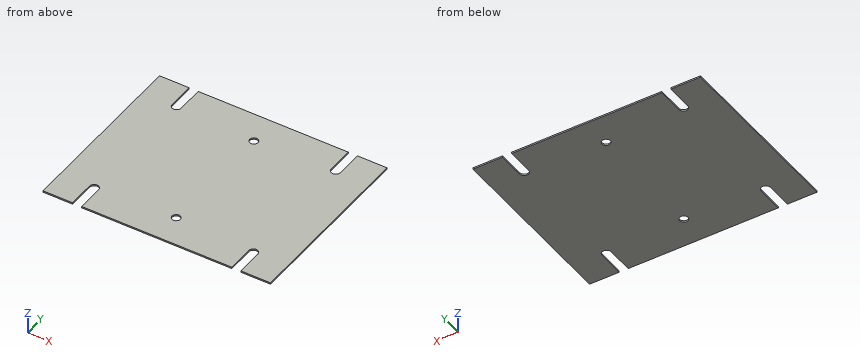
from build123d import *

# Parameters (mm, degrees)
SKETCH1_R               = 5.5
SKETCH1_R_2             = 3.25
BOSS_EXTRUDE1_DEPTH     = 2
CUT_EXTRUDE1_DEPTH      = 319.029152687
CUT_EXTRUDE1_DEPTH_BACK = 319.029152687
SKETCH2_W               = 30
SKETCH2_H               = 70
CUT_EXTRUDE2_DEPTH      = 319.029152687
CUT_EXTRUDE2_DEPTH_BACK = 319.029152687
SKETCH3_W               = 30
SKETCH3_H               = 70


with BuildPart() as part:
    # Sketch1 → Boss-Extrude1 (new body)
    with BuildSketch(Plane.XY):
        with BuildLine():
            Line((68.948821818, -26.633764286), (98.948821818, -26.633764286))
            Line((98.948821818, -26.633764286), (98.948821818, -96.633764286))
            Line((98.948821818, -96.633764286), (68.948821818, -96.633764286))
            Line((68.948821818, -96.633764286), (68.948821818, -181.633764286))
            Line((68.948821818, -181.633764286), (29.948821818, -181.633764286))
            Line((29.948821818, -181.633764286), (29.948821818, -146.633764286))
            ThreePointArc((29.948821818, -146.633764286), (23.948821818, -140.633764286), (17.948821818, -146.633764286))
            Line((17.948821818, -146.633764286), (17.948821818, -181.633764286))
            Line((17.948821818, -181.633764286), (-180.051178182, -181.633764286))
            Line((-180.051178182, -181.633764286), (-180.051178182, -146.633764286))
            ThreePointArc((-180.051178182, -146.633764286), (-186.051178182, -140.633764286), (-192.051178182, -146.633764286))
            Line((-192.051178182, -146.633764286), (-192.051178182, -181.633764286))
            Line((-192.051178182, -181.633764286), (-231.051178182, -181.633764286))
            Line((-231.051178182, -181.633764286), (-231.051178182, -100.179856115))
            Line((-231.051178182, -100.179856115), (-261.051178182, -100.179856115))
            Line((-261.051178182, -100.179856115), (-261.051178182, -30.179856115))
            Line((-261.051178182, -30.179856115), (-231.051178182, -30.179856115))
            Line((-231.051178182, -30.179856115), (-231.051178182, 58.366235714))
            Line((-231.051178182, 58.366235714), (-192.051178182, 58.366235714))
            Line((-192.051178182, 58.366235714), (-192.051178182, 23.366235714))
            ThreePointArc((-192.051178182, 23.366235714), (-186.051178182, 17.366235714), (-180.051178182, 23.366235714))
            Line((-180.051178182, 23.366235714), (-180.051178182, 58.366235714))
            Line((-180.051178182, 58.366235714), (17.948821818, 58.366235714))
            Line((17.948821818, 58.366235714), (17.948821818, 23.366235714))
            ThreePointArc((17.948821818, 23.366235714), (23.948821818, 17.366235714), (29.948821818, 23.366235714))
            Line((29.948821818, 23.366235714), (29.948821818, 58.366235714))
            Line((29.948821818, 58.366235714), (68.948821818, 58.366235714))
            Line((68.948821818, 58.366235714), (68.948821818, -26.633764286))
        make_face()
        with Locations((-81.051178182, -141.633764286)):
            Circle(SKETCH1_R, mode=Mode.SUBTRACT)
        with Locations((-81.051178182, 18.366235714)):
            Circle(SKETCH1_R, mode=Mode.SUBTRACT)
        with Locations((83.948821818, -61.633764286)):
            Circle(SKETCH1_R_2, mode=Mode.SUBTRACT)
        with Locations((-246.051178182, -65.179856115)):
            Circle(SKETCH1_R_2, mode=Mode.SUBTRACT)
    extrude(amount=BOSS_EXTRUDE1_DEPTH)

    # Sketch2 → Cut-Extrude1 (cut, two sides: drawn at the far end of the back side and taken through both)
    with BuildSketch(Plane.XY.offset(2).offset(-CUT_EXTRUDE1_DEPTH_BACK)):
        with Locations((83.948821818, -61.633764286)):
            Rectangle(SKETCH2_W, SKETCH2_H)
    extrude(amount=CUT_EXTRUDE1_DEPTH + CUT_EXTRUDE1_DEPTH_BACK, mode=Mode.SUBTRACT)

    # Sketch3 → Cut-Extrude2 (cut, two sides: drawn at the far end of the back side and taken through both)
    with BuildSketch(Plane.XY.offset(2).offset(-CUT_EXTRUDE2_DEPTH_BACK)):
        with Locations((-246.051178182, -65.179856115)):
            Rectangle(SKETCH3_W, SKETCH3_H)
    extrude(amount=CUT_EXTRUDE2_DEPTH + CUT_EXTRUDE2_DEPTH_BACK, mode=Mode.SUBTRACT)


solid = part.part
Input: part model. Units: mm. Frame: model coordinates. Round coordinates to 2 decimals unless told otherwise and drop trailing zeros. Order: outer loops, then holes, each group sorted by start corner. A loop starts at its lowest first (then second) coordinate and runs counter-clockwise, first axis right, second up. Notation, with made-up numbers: (-39.5, 40) - (11.5, 40) arc R12 cw to (11.5, 51) - close; hole circle Ø11 at (60, 12.5). An arc over 180 degrees is marked (long way). Answer as a JSON object with one key per item and string values. Group by question number.
(1) Pin query (flat end, axial travel): P1, Ø10, axis at x = -81.05, y = 18.37, coming from the -Z side. Return the tip coordinate at first contact, or that it passes through.
(2) Material intervals for probe 1 along X at (y, z) = (46, 0.2); probe 2 along Y at (x, z) = (-77.5, 0.4); probe 3 along X at (y, z) = (16, 1.2), sorted ascending. Write a range as from..to.
(3) Cut plane A-A (y = 27.5). Return loops of the section in (x, z).
(4) Cut plane B-B (z = 0.3). Return loops of the section in (x, y).
Here are the results:
{
 "1": {"P1": "passes through"},
 "2": {"probe 1": "x = -231.05..-192.05, -180.05..17.95, 29.95..68.95", "probe 2": "y = -181.63..-145.83, -137.43..14.17, 22.57..58.37", "probe 3": "x = -231.05..-86.02, -76.09..68.95"},
 "3": {"outline": "(-231.05, 0) - (-192.05, 0) - (-192.05, 2) - (-231.05, 2) - close; (-180.05, 0) - (17.95, 0) - (17.95, 2) - (-180.05, 2) - close; (29.95, 0) - (68.95, 0) - (68.95, 2) - (29.95, 2) - close"},
 "4": {"outline": "(-231.05, -181.63) - (-192.05, -181.63) - (-192.05, -146.63) arc R6 cw to (-180.05, -146.63) - (-180.05, -181.63) - (17.95, -181.63) - (17.95, -146.63) arc R6 cw to (29.95, -146.63) - (29.95, -181.63) - (68.95, -181.63) - (68.95, 58.37) - (29.95, 58.37) - (29.95, 23.37) arc R6 cw to (17.95, 23.37) - (17.95, 58.37) - (-180.05, 58.37) - (-180.05, 23.37) arc R6 cw to (-192.05, 23.37) - (-192.05, 58.37) - (-231.05, 58.37) - close; hole circle Ø11 at (-81.05, -141.63); hole circle Ø11 at (-81.05, 18.37)"}
}
